from build123d import *

# Parameters (mm, degrees)
SKETCH1_R            = 1.6
BOSS_EXTRUDE1_DEPTH  = 2.95
FILLET1_R            = 5
M3_CLEARANCE_HOLE3_D = 3.2
LPATTERN3_COUNT      = 7
LPATTERN3_PITCH      = 10
LPATTERN3_COUNT_DIR2 = 11
LPATTERN3_PITCH_DIR2 = 10


with BuildPart() as part:
    # Sketch1 → Boss-Extrude1 (new body)
    with BuildSketch(Plane.XY):
        with BuildLine():
            Line((3.56, -29.301188946), (3.56, -55))
            Line((3.56, -55), (80, -55))
            Line((80, -55), (80, 55))
            Line((80, 55), (3.56, 55))
            Line((3.56, 55), (3.56, 29.301188946))
            ThreePointArc((3.56, 29.301188946), (11.789075932, 31.144059076), (16.53, 24.17))
            Line((16.53, 24.17), (16.53, -24.17))
            ThreePointArc((16.53, -24.17), (11.789075932, -31.144059076), (3.56, -29.301188946))
        make_face()
        with Locations((9.03, -48.875)):
            Circle(SKETCH1_R, mode=Mode.SUBTRACT)
        with Locations((73.525, -48.875)):
            Circle(SKETCH1_R, mode=Mode.SUBTRACT)
        with Locations((9.03, 48.875)):
            Circle(SKETCH1_R, mode=Mode.SUBTRACT)
        with Locations((73.525, 48.875)):
            Circle(SKETCH1_R, mode=Mode.SUBTRACT)
    extrude(amount=BOSS_EXTRUDE1_DEPTH)

    # Fillet1
    fillet1_edges = [part.edges().sort_by_distance(p)[0] for p in [
        (3.56, 29.301188946, 1.475),
        (3.56, -29.301188946, 1.475),
    ]]
    fillet(fillet1_edges, radius=FILLET1_R)

    # M3 Clearance Hole3 (through all)
    with Locations(Plane(origin=(0, 0, 0), x_dir=(-1, 0, 0), z_dir=(0, 0, -1))):
        with Locations((-15, -50)):
            m3_clearance_hole3 = Hole(M3_CLEARANCE_HOLE3_D / 2)

    # LPattern3: M3 Clearance Hole3 7 × 11, 9 skipped
    with Locations(*[(i * LPATTERN3_PITCH, j * LPATTERN3_PITCH_DIR2, 0) for i in range(LPATTERN3_COUNT) for j in range(LPATTERN3_COUNT_DIR2) if (i, j) not in ((0, 0), (0, 2), (0, 3), (0, 4), (0, 5), (0, 6), (0, 7), (0, 8), (6, 0), (6, 10))]):
        add(m3_clearance_hole3, mode=Mode.SUBTRACT)


solid = part.part
The listing builds one solid part. Answer for the finished solid, in the listing's coordinates (mm). Round coordinates to 2 decimals unless told otherwise and drop trailing zeros. Write each loop counter-clockwise with the first axis right and the second up, starting at its lowest first coordinate (ties: lowest second). Pieces come first, ordered by that corner, then holes. Notation, with made-up numbers: M 81,-21 L 124,-21 A19 ccw 124,14 Z; hole C 52,-16.5 d11. An arc over 180 degrees is marked long. Write each question's results on one line, items separated by ' | '. Start each with the question number.
Item 1: A cutting plane is placed at A-A on y = 40. State how many separate pieces and enclosed holes the cut face has, and give its area (3 significant figures).
Item 2: For a pull along Y with two mould halves and no side action, classify faces 1 (the face through (42, 55, 1)), 2 (the face through (66.526, 20.481, 1.496)) as pulls with the +Y half, pulls with the -Y half, needs draft (parallel to the pull), parting line crosses it, or undercut.
Item 3: A cutting plane is placed at C-C on x = 15. Write down the section's boundary in (y, z).
Item 4: A cutting plane is placed at B-B on y = -30. Write down the section's boundary in (x, z), and give its area (3 significant figures).
Item 5: Straight lines are drawn through the part: L1, parallel to Y at x = 9.03, z = 1.1 (3 decimals); L2, parallel to X at y = 48, z = 1.5; L3, parallel to Y at x = 15, z = 0.7. For each, find the intervals that lie inside material, in ascending order. Write a range as [from, to].
Check sheet entries:
1) separate pieces: 8 | enclosed holes: 0 | area: 159 mm²
2) face 1: pulls with the +Y half | face 2: undercut
3) outline: M -55,0 L -51.6,0 L -51.6,2.95 L -55,2.95 Z; M -48.4,0 L -41.6,0 L -41.6,2.95 L -48.4,2.95 Z; M -38.4,0 L -28.71,0 L -28.71,2.95 L -38.4,2.95 Z; M 28.71,0 L 38.4,0 L 38.4,2.95 L 28.71,2.95 Z; M 41.6,0 L 48.4,0 L 48.4,2.95 L 41.6,2.95 Z; M 51.6,0 L 55,0 L 55,2.95 L 51.6,2.95 Z
4) outline: M 13.75,0 L 23.4,0 L 23.4,2.95 L 13.75,2.95 Z; M 26.6,0 L 33.4,0 L 33.4,2.95 L 26.6,2.95 Z; M 36.6,0 L 43.4,0 L 43.4,2.95 L 36.6,2.95 Z; M 46.6,0 L 53.4,0 L 53.4,2.95 L 46.6,2.95 Z; M 56.6,0 L 63.4,0 L 63.4,2.95 L 56.6,2.95 Z; M 66.6,0 L 73.4,0 L 73.4,2.95 L 66.6,2.95 Z; M 76.6,0 L 80,0 L 80,2.95 L 76.6,2.95 Z | area: 139 mm²
5) L1: [-55, -50.475], [-47.275, -31.67], [31.67, 47.275], [50.475, 55] | L2: [3.56, 7.69], [10.37, 72.19], [74.86, 80] | L3: [-55, -51.6], [-48.4, -41.6], [-38.4, -28.71], [28.71, 38.4], [41.6, 48.4], [51.6, 55]
